from build123d import *

# Parameters (mm, degrees)
CYLINDER_R     = 2.5
CYLINDER_DEPTH = 20
BOX_W          = 7.5
BOX_H          = 20
BOX_DEPTH      = 4.8
BOX001_W       = 20
BOX001_H       = 29
BOX001_DEPTH   = 7
FILLET_R       = 2
FILLET001_R    = 2
CHAMFER_SIZE   = 0.5


with BuildPart() as cilindro:
    # Cylinder → Cylinder (new body)
    with BuildSketch(Plane(origin=(0, -10, -10), x_dir=(1, 0, 0), z_dir=(0, 0, 1))):
        Circle(CYLINDER_R)
    extrude(amount=CYLINDER_DEPTH)


with BuildPart() as obj1:
    # Box → Box (new body)
    with BuildSketch(Plane(origin=(-3.75, 0, -1), x_dir=(1, 0, 0), z_dir=(0, 0, 1))):
        with Locations((3.75, 10)):
            Rectangle(BOX_W, BOX_H)
    extrude(amount=BOX_DEPTH)


with BuildPart() as chamfer_body:
    # Box001 → Box001 (new body)
    with BuildSketch(Plane(origin=(-10, -20, 0), x_dir=(1, 0, 0), z_dir=(0, 0, 1))):
        with Locations((10, 14.5)):
            Rectangle(BOX001_W, BOX001_H)
    extrude(amount=BOX001_DEPTH)

    # Cut: cut obj1
    add(obj1.part, mode=Mode.SUBTRACT)

    # Cut001: cut Cilindro
    add(cilindro.part, mode=Mode.SUBTRACT)

    # Fillet
    fillet_edges = [chamfer_body.edges().sort_by_distance(p)[0] for p in [
        (-10, -20, 3.5),
        (10, -20, 3.5),
    ]]
    fillet(fillet_edges, radius=FILLET_R)

    # Fillet001
    fillet001_edges = [chamfer_body.edges().sort_by_distance(p)[0] for p in [
        (-10, -4.5, 7),
    ]]
    fillet(fillet001_edges, radius=FILLET001_R)

    # Chamfer
    chamfer_edges = [chamfer_body.edges().sort_by_distance(p)[0] for p in [
        (-2.5, -10, 7),
    ]]
    chamfer(chamfer_edges, length=CHAMFER_SIZE)


solid = chamfer_body.part
Model file for the job. Use its own axes, mm. A direction names the side the tool comes from. Round coordinates to 2 decimals unless told otherwise and drop trailing zeros. Loops run counter-clockwise (first coordinate to the right, second up) from the corner with the lowest first, then second, coordinate; pieces in that order, holes last. Notation, with made-up numbers: (20, -33) -> (77, -33) arc R27 ccw to (77, -6) -> close; hole circle Ø10 at (34.25, 75). An arc over 180 degrees is marked (long way). Answer as CSV lines item,"result". Start each with the question number.
1) Slice it at B-B (y = -10). List the corners of the cut face in (x, z), plus the area to 3 significant figures.
2) Mould opens along Y. For faces 1 (the face through (0, 0, 2)), 2 (the face through (-0.54, -12.44, 3.2)), 3 (the face through (0, 5, 3.8)), 4 (the face through (0, -20, 2)) say: +Y half, -Y half, draft (parallel to the pull), parting line (faces both ways), or undercut.
3) Probe line 1 along Y through (x, z) = (0, 3.75); line 2 along X through (y, z) = (-10, 1.75); line 3 along X through (y, z) = (2.25, 3.75). List the from-to ranges inside material, lowest first.
4) Pin check, flat tips, straight feed: P1, Ø6, axis at x = 0, y = -10, coming from the -Z side; P2, Ø4, axis at x = 1, y = 3.5, coming from the -Z side. Stop position of each tip, or through.
5) Tool access for faces 5 (the face through (-3.75, 4, 2)), 6 (the face through (-9.43, -4.31, 6.4)): list every direction of +Z, -Z, +X, -X, +Y, -Y with a clear straight run to the whole face (end or side of a thin tool).
6) Slice it at A-A (x = 0). List the corners of the cut face in (y, z), plus the area to 3 significant figures.
7) Slice it at C-C (z = 1.75). List the corners of the cut face in (x, y).
8) Slice it at D-D (z = 4.5). List the corners of the cut face in (x, y), plus the area to 3 significant figures.
Filled in:
1,outline,"(-10, 0) -> (-2.5, 0) -> (-2.5, 6.5) -> (-3, 7) -> (-8, 7) arc R2 ccw to (-10, 5) -> close; (2.5, 0) -> (10, 0) -> (10, 5) arc R2 ccw to (8, 7) -> (3, 7) -> (2.5, 6.5) -> close"
1,area,"103 mm2"
2,face 1,"+Y half"
2,face 2,"undercut"
2,face 3,"draft"
2,face 4,"-Y half"
3,line 1,"y = -20 to -12.5, -7.5 to 0"
3,line 2,"x = -10 to -2.5, 2.5 to 10"
3,line 3,"x = -10 to -3.75, 3.75 to 10"
4,P1,"stops at z = 0"
4,P2,"stops at z = 3.8"
5,face 5,"-Z, +Y"
5,face 6,"+Z, -X, +Y, -Y"
6,outline,"(-20, 0) -> (-12.5, 0) -> (-12.5, 6.5) -> (-13, 7) -> (-18, 7) arc R2 ccw to (-20, 5) -> close; (-7.5, 0) -> (0, 0) -> (0, 3.8) -> (9, 3.8) -> (9, 7) -> (-7, 7) -> (-7.5, 6.5) -> close"
6,area,"133 mm2"
7,outline,"(-10, -18) arc R2 ccw to (-8, -20) -> (8, -20) arc R2 ccw to (10, -18) -> (10, 9) -> (3.75, 9) -> (3.75, 0) -> (-3.75, 0) -> (-3.75, 9) -> (-10, 9) -> close; hole circle Ø5 at (0, -10)"
8,outline,"(-10, -18) arc R2 ccw to (-8, -20) -> (8, -20) arc R2 ccw to (10, -18) -> (10, 9) -> (-10, 9) -> close; hole circle Ø5 at (0, -10)"
8,area,"559 mm2"
